```python
from build123d import *

# Parameters (mm, degrees)
SKETCH1_W           = 84
SKETCH1_H           = 55
BOSS_EXTRUDE1_DEPTH = 8
SKETCH2_W           = 3.987273362
SKETCH2_H           = 3.987273362
BOSS_EXTRUDE2_DEPTH = 1.5
SKETCH3_W           = 3.99
SKETCH3_H           = 3.99
BOSS_EXTRUDE3_DEPTH = 1.5
SKETCH6_W           = 3.99
SKETCH6_H           = 3.99
BOSS_EXTRUDE4_DEPTH = 1.5
SKETCH7_W           = 3.99
SKETCH7_H           = 3.99
BOSS_EXTRUDE5_DEPTH = 1.5
SKETCH10_R          = 6
BOSS_EXTRUDE6_DEPTH = 2.7


with BuildPart() as part:
    # Sketch1 → Boss-Extrude1 (new body)
    with BuildSketch(Plane(origin=(0, 0, 0), x_dir=(1, 0, 0), z_dir=(0, 1, 0))):
        Rectangle(SKETCH1_W, SKETCH1_H)
    extrude(amount=BOSS_EXTRUDE1_DEPTH)

    # Sketch2 → Boss-Extrude2 (add)
    with BuildSketch(Plane(origin=(0, -0.439186924, 27.5), x_dir=(1, 0, 0), z_dir=(0, 0, 1))):
        with Locations((-30.884576243, 4.455349568)):
            Rectangle(SKETCH2_W, SKETCH2_H)
    extrude(amount=BOSS_EXTRUDE2_DEPTH)

    # Sketch3 → Boss-Extrude3 (add)
    with BuildSketch(Plane(origin=(0, -0.590315395, 27.5), x_dir=(1, 0, 0), z_dir=(0, 0, 1))):
        with Locations((31.62769067, 4.58925653)):
            Rectangle(SKETCH3_W, SKETCH3_H)
    extrude(amount=BOSS_EXTRUDE3_DEPTH)

    # Sketch6 → Boss-Extrude4 (add)
    with BuildSketch(Plane(origin=(42, 0.101407509, -1.505913579), x_dir=(0, 0, -1), z_dir=(1, 0, 0))):
        with Locations((-18.317394251, 4.044008008)):
            Rectangle(SKETCH6_W, SKETCH6_H)
    extrude(amount=BOSS_EXTRUDE4_DEPTH)

    # Sketch7 → Boss-Extrude5 (add)
    with BuildSketch(Plane(origin=(42, -0.062003659, -3.114914247), x_dir=(0, 0, -1), z_dir=(1, 0, 0))):
        with Locations((13.283568203, 4.150096741)):
            Rectangle(SKETCH7_W, SKETCH7_H)
    extrude(amount=BOSS_EXTRUDE5_DEPTH)

    # Sketch10 → Boss-Extrude6 (add)
    with BuildSketch(Plane(origin=(0, 8, 0), x_dir=(1, 0, 0), z_dir=(0, 1, 0))):
        with Locations((-32, 0)):
            Circle(SKETCH10_R)
    extrude(amount=BOSS_EXTRUDE6_DEPTH)


solid = part.part
```
Geometry: final body of the model. Coordinates: model frame, mm. Give positions to 0.01 mm unless a question says otherwise; leave off trailing zeros. Write each loop counter-clockwise with the first axis right and the second up, starting at its lowest first coordinate (ties: lowest second). Pieces come first, ordered by that corner, then holes.
1. Pin query (flat end, axial travel): P1, Ø6, axis at y = 2, z = 12, coming from the +X side; P2, Ø4, axis at x = 7, y = 2.5, coming from the +Z side; P3, Ø6, axis at x = -18, z = -21.5, coming from the +Y side; P4, Ø1.6, axis at x = -31, z = 28.5, coming from the +Y side. Return the tip coordinate at first contact, or that it passes through.
2. Section query C-C, the plane x = -32. Return loops of the section in (y, z), then the cut area to 3 significant figures.
3. Section query A-A, the plane z = 0. Return loops of the section in (x, y), then the cut area to 3 significant figures.
4. Section query D-D, the plane y = 9.5. Return loops of the section in (x, z).
5. Line query: probe 1 along Y at (x, z) = (-2, -15.5); probe 2 along X at (y, z) = (2.5, -5); probe 3 along Z at (x, y) = (-6, 6.5). Output: solid intervals per line, ascending.
6. Draft query along X for faces 1 (the flat face through (-1, 4, 27.5)), 2 (the flat face through (-42, 4, 0)), 3 (the flat face through (-1, 8, 0)), 4 (the cylindrical face through (-38, 9, 0)). Return one class per face: released by +X, released by -X, zero draft, split by the parting line, or undercut.
7. Section query B-B, the plane x = 30.5. Return loops of the section in (y, z), then the cut area to 3 significant figures.
Computed:
1. P1: stops at x = 43.5
1. P2: stops at z = 27.5
1. P3: stops at y = 8
1. P4: stops at y = 6.01
2. outline: (0, -27.5) - (8, -27.5) - (8, -6) - (10.7, -6) - (10.7, 6) - (8, 6) - (8, 27.5) - (6.01, 27.5) - (6.01, 29) - (2.02, 29) - (2.02, 27.5) - (0, 27.5) - close
2. area: 478 mm2
3. outline: (-42, 0) - (42, 0) - (42, 8) - (-26, 8) - (-26, 10.7) - (-38, 10.7) - (-38, 8) - (-42, 8) - close
3. area: 704 mm2
4. outline: circle Ø12 at (-32, 0)
5. probe 1: y = 0 to 8
5. probe 2: x = -42 to 42
5. probe 3: z = -27.5 to 27.5
6. face 1: undercut
6. face 2: released by -X
6. face 3: zero draft
6. face 4: split by the parting line
7. outline: (0, -27.5) - (8, -27.5) - (8, 27.5) - (5.99, 27.5) - (5.99, 29) - (2, 29) - (2, 27.5) - (0, 27.5) - close
7. area: 446 mm2
